```python
from build123d import *

# Parameters (mm, degrees)
F0_W     = 260
F0_H     = 60
F1_DEPTH = 3
F2_R     = 2.25
F3_DEPTH = 3.001
F4_R     = 10


with BuildPart() as f1:
    # F0 (on Front) → F1 (new body)
    with BuildSketch(Plane.XZ):
        Rectangle(F0_W, F0_H)
    extrude(amount=F1_DEPTH)

    # F2 (on face) → F3 (cut, through all)
    with BuildSketch(Plane.XZ.offset(3)):
        with Locations((-120, 20)):
            Circle(F2_R)
        with Locations((-120, -20)):
            Circle(F2_R)
        with Locations((-88, 20)):
            Circle(F2_R)
        with Locations((-88, -20)):
            Circle(F2_R)
        with Locations((88, 20)):
            Circle(F2_R)
        with Locations((120, 20)):
            Circle(F2_R)
        with Locations((120, -20)):
            Circle(F2_R)
        with Locations((88, -20)):
            Circle(F2_R)
    extrude(amount=-F3_DEPTH, mode=Mode.SUBTRACT)

    # F4
    f4_edges = [f1.edges().sort_by_distance(p)[0] for p in [
        (-130, -1.5, 30),
        (-130, -1.5, -30),
        (130, -1.5, -30),
        (130, -1.5, 30),
    ]]
    fillet(f4_edges, radius=F4_R)


solid = f1.part
```
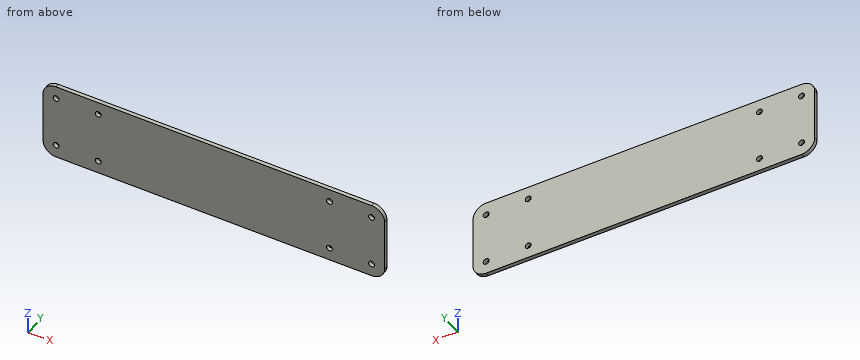
For this review, take the finished solid that the model builds, in its own axes (mm). Give positions to 0.01 mm unless a question says otherwise; leave off trailing zeros. Write each loop counter-clockwise with the first axis right and the second up, starting at its lowest first coordinate (ties: lowest second). Pieces come first, ordered by that corner, then holes. Notation, with made-up numbers: M -31.75,33 L -18.75,33 A19 ccw -18.75,66 Z; hole C 30.5,31.25 d2. An arc over 180 degrees is marked long. Answer as a JSON object with one key per item and string values. Group by question number.
Item 1: Consider section A-A on x = -88. Write out the cut boundary in (y, z).
Item 2: For pin 1 Ø3.5 at (x, z) = (120, -20) entering from +Y, flat-tipped, find the tip position at first contact; note if it passes through.
Item 3: For probe 1 along Z at (x, y) = (120, -1.7); probe 2 along Z at (x, y) = (87, -0.4); probe 3 along X at (y, z) = (-1.4, 25.5), list the stretches that pass through material, from the lowest coordinate up. Write a range as [from, to].
Check result:
{
 "1": {"outline": "M -3,-30 L 0,-30 L 0,-22.25 L -3,-22.25 Z; M -3,-17.75 L 0,-17.75 L 0,17.75 L -3,17.75 Z; M -3,22.25 L 0,22.25 L 0,30 L -3,30 Z"},
 "2": {"pin 1": "passes through"},
 "3": {"probe 1": "z = [-30, -22.25], [-17.75, 17.75], [22.25, 30]", "probe 2": "z = [-30, -22.02], [-17.98, 17.98], [22.02, 30]", "probe 3": "x = [-128.35, 128.35]"}
}
